```python
from build123d import *

# Parameters (mm, degrees)
SKETCH3_W           = 0.8
SKETCH3_H           = 4.75
BOSS_EXTRUDE1_DEPTH = 9


with BuildPart() as part:
    # Sketch1 → Revolve2 (revolve)
    with BuildSketch(Plane.XY, mode=Mode.PRIVATE) as revolve2_sk:
        with BuildLine():
            Line((0, -13.24200419), (-9.5, -13.24200419))
            Line((-9.5, -13.24200419), (-9.5, 0.9180652))
            Line((-9.5, 0.9180652), (-11.5, 0.9180652))
            Line((-11.5, 0.9180652), (-11.5, 2.69389815))
            Line((-11.5, 2.69389815), (-9.59273849, 3.99115987))
            Line((-9.59273849, 3.99115987), (-10.921099291, 4.332198136))
            ThreePointArc((-10.921099291, 4.332198136), (-11.482083746, 5.119970296), (-10.800193426, 5.805764819))
            Line((-10.800193426, 5.805764819), (-8.297971346, 6.025460413))
            Line((-8.297971346, 6.025460413), (-8.297971346, 6.184171242))
            Line((-8.297971346, 6.184171242), (-10.316863696, 6.794381901))
            ThreePointArc((-10.316863696, 6.794381901), (-10.83463658, 7.361906816), (-10.581495802, 8.087229527))
            Line((-10.581495802, 8.087229527), (-9.280818948, 9.176830883))
            Line((-9.280818948, 9.176830883), (0, 9.176830883))
            Line((0, 9.176830883), (0, -13.24200419))
        make_face()
    revolve(revolve2_sk.sketch.rotate(Axis((0, 40.42841221, 0), (0, -1, 0)), 270), axis=Axis((0, 40.42841221, 0), (0, -1, 0)))

    # Sketch2 → Revolve3 (revolve)
    with BuildSketch(Plane.XY, mode=Mode.PRIVATE) as revolve3_sk:
        with BuildLine():
            Line((0, 9.176830883), (-9.280818948, 9.176830883))
            ThreePointArc((-9.280818948, 9.176830883), (-4.681726791, 10.106381279), (0, 10.4180652))
            Line((0, 10.4180652), (0, 9.176830883))
        make_face()
    revolve(revolve3_sk.sketch.rotate(Axis((0, 15.762950143, 0), (0, -1, 0)), 270), axis=Axis((0, 15.762950143, 0), (0, -1, 0)))

    # Sketch3 → Boss-Extrude1 (add)
    with BuildSketch(Plane.XZ.offset(13.24200419)):
        with Locations((-4.875927863, 3.979511683)):
            Rectangle(SKETCH3_W, SKETCH3_H)
        with Locations((4.875927863, 3.979511683)):
            Rectangle(SKETCH3_W, SKETCH3_H)
        with Locations((4.875927863, -3.979511683)):
            Rectangle(SKETCH3_W, SKETCH3_H)
        with Locations((-4.875927863, -3.979511683)):
            Rectangle(SKETCH3_W, SKETCH3_H)
    extrude(amount=BOSS_EXTRUDE1_DEPTH)


solid = part.part
```
Read the model definition and answer for the solid it produces. Units are mm, in the model's axes. A direction names the side the tool comes from. Round coordinates to 2 decimals unless told otherwise and drop trailing zeros. Write each loop counter-clockwise with the first axis right and the second up, starting at its lowest first coordinate (ties: lowest second). Pieces come first, ordered by that corner, then holes. Notation, with made-up numbers: M 26,-34 L 75,-34 A33 cw 75,-3 Z; hole C 37.25,60.5 d2. An arc over 180 degrees is marked long. One line per item, written item: value.
Q1. For a pull along X with two mould halves and no side action, classify faces 1 (the flat face through (5.276, -18, -4)), 2 (the flat face through (4.476, -18, -4)), 3 (the cylindrical face through (-9.7, 1.82, 6.18)), 4 (the flat face through (4.476, -18, 4)) as +X half, -X half, draft (parallel to the pull), parting line (faces both ways), or undercut.
Data:
face 1: +X half
face 2: undercut
face 3: parting line
face 4: undercut
Q2. Find section C-C on z = 0. Write down the section's boundary in (x, y), plus the area to 3 significant figures.
Data:
outline: M -11.5,0.92 L -9.5,0.92 L -9.5,-13.24 L 9.5,-13.24 L 9.5,0.92 L 11.5,0.92 L 11.5,2.69 L 9.59,3.99 L 10.92,4.33 A0.75 ccw 10.8,5.81 L 8.3,6.03 L 8.3,6.18 L 10.32,6.79 A0.75 ccw 10.58,8.09 L 9.28,9.18 A35.32 ccw -9.28,9.18 L -10.58,8.09 A0.75 ccw -10.32,6.79 L -8.3,6.18 L -8.3,6.03 L -10.8,5.81 A0.75 ccw -10.92,4.33 L -9.59,3.99 L -11.5,2.69 Z
area: 461 mm2
Q3. Find section A-A on y = -17. Write down the section's boundary in (x, z).
Data:
outline: M -5.28,-6.35 L -4.48,-6.35 L -4.48,-1.6 L -5.28,-1.6 Z; M -5.28,1.6 L -4.48,1.6 L -4.48,6.35 L -5.28,6.35 Z; M 4.48,-6.35 L 5.28,-6.35 L 5.28,-1.6 L 4.48,-1.6 Z; M 4.48,1.6 L 5.28,1.6 L 5.28,6.35 L 4.48,6.35 Z
Q4. Flat-ended cylindrical pins translate along their axes: pin 1 Ø2.5 at (y, z) = (-19, -3) entering from +X; pin 2 Ø1.4 at (y, z) = (-20, 4.5) entering from -X; pin 3 Ø0.9 at (x, y) = (5, -18) entering from -Z. Find the tip coordinate at first contact, or state that the pin passes through.
Data:
pin 1: x = 5.28
pin 2: x = -5.28
pin 3: z = -6.35
Q5. Find section B-B on x = 0. Write down the section's boundary in (y, z), plus the area to 3 significant figures.
Data:
outline: M -13.24,-9.5 L 0.92,-9.5 L 0.92,-11.5 L 2.69,-11.5 L 3.99,-9.59 L 4.33,-10.92 A0.75 ccw 5.81,-10.8 L 6.03,-8.3 L 6.18,-8.3 L 6.79,-10.32 A0.75 ccw 8.09,-10.58 L 9.18,-9.28 A35.32 ccw 9.18,9.28 L 8.09,10.58 A0.75 ccw 6.79,10.32 L 6.18,8.3 L 6.03,8.3 L 5.81,10.8 A0.75 ccw 4.33,10.92 L 3.99,9.59 L 2.69,11.5 L 0.92,11.5 L 0.92,9.5 L -13.24,9.5 Z
area: 461 mm2
Q6. Which of the six approach directions +Z, -Z, +X, -X, +Y, -Y give full straight-line access (tool end or side, diameter ignored) to faces 5 (the flat face through (-5, -18, -6.355)), 6 (the flat face through (5.276, -18, 4)), 7 (the flat face through (5, -18, 1.605)), 8 (the flat face through (-5.276, -18, 4)), 9 (the flat face through (-4.476, -18, -4))?
Data:
face 5: -Z, +X, -X, -Y
face 6: +Z, -Z, +X, -Y
face 7: +X, -X, -Y
face 8: +Z, -Z, -X, -Y
face 9: +Z, -Z, -Y
Q7. Straight lines are drawn through the part: line 1 (Y direction, x = 3.5, z = 9.75); line 2 (Y direction, x = 10, z = -1.25); line 3 (X direction, y = 1, z = 0.5). For each, find the intervals that lie inside material, in ascending order. Write a range as [from, to].
Data:
line 1: [0.92, 3.47], [4.19, 5.84], [6.81, 8.27]
line 2: [0.92, 3.66], [4.12, 5.87], [6.72, 8.51]
line 3: [-11.49, 11.49]
Q8. Find section D-D on y = -6. Write down the section's boundary in (x, z).
Data:
outline: C 0,0 d19
